Study the drawing (mm; zero at the part's minimum x, y, z) and answer. A direction names the side the tool comes from. Coordinates: 2 decimals unless noted, no trailing zeros. Order: outer loops, then holes, each group sorted by start corner. A loop starts at its lowest first (then second) coordinate and runs counter-clockwise, first axis right, second up.
1. A tool of negligible diameter and unlimited length cuts with its end or side. For the marked faces 1, 2, 3 and 4, from which of +Z, -Z, +X, -X, +Y, -Y can it reach the whole face along a straight path? Write none if from no direction.
2. The part is cut by section C-C, the plane x = 22. Give the vertices of the cut face in (y, z).
3. The part is cut by section A-A, the plane y = 2.5. Give the vertices of the cut face in (x, z), then the cut area to 3 significant figures.
4. Find the intervals of material crossed by probe 1 along X at (y, z) = (1.15, 25); probe 2 along Z at (x, y) = (10.05, 11), in increasing order.
5. Flat-ended cylindrical pins translate along their axes: pin 1 Ø8 at (x, y) = (27, 12.5) entering from -Z; pin 2 Ø2 at (x, y) = (5.5, 9.5) entering from +Z; pin 3 Ø2 at (y, z) = (10.5, 15.5) entering from +X. Find the tip coordinate at first contact, or state that the pin passes through.
6. The part is cut by section B-B, the plane z = 25. Give the vertices of the cut face in (x, y).
7. The part is cut by section D-D, the plane z = 18.5. Give the vertices of the cut face in (x, y).
8. Determine the mould class of the marked faces 5, 6, 7 and 8 for opening direction X: +X half, -X half, draft (parallel to the pull), parting line (faces both ways), or undercut.
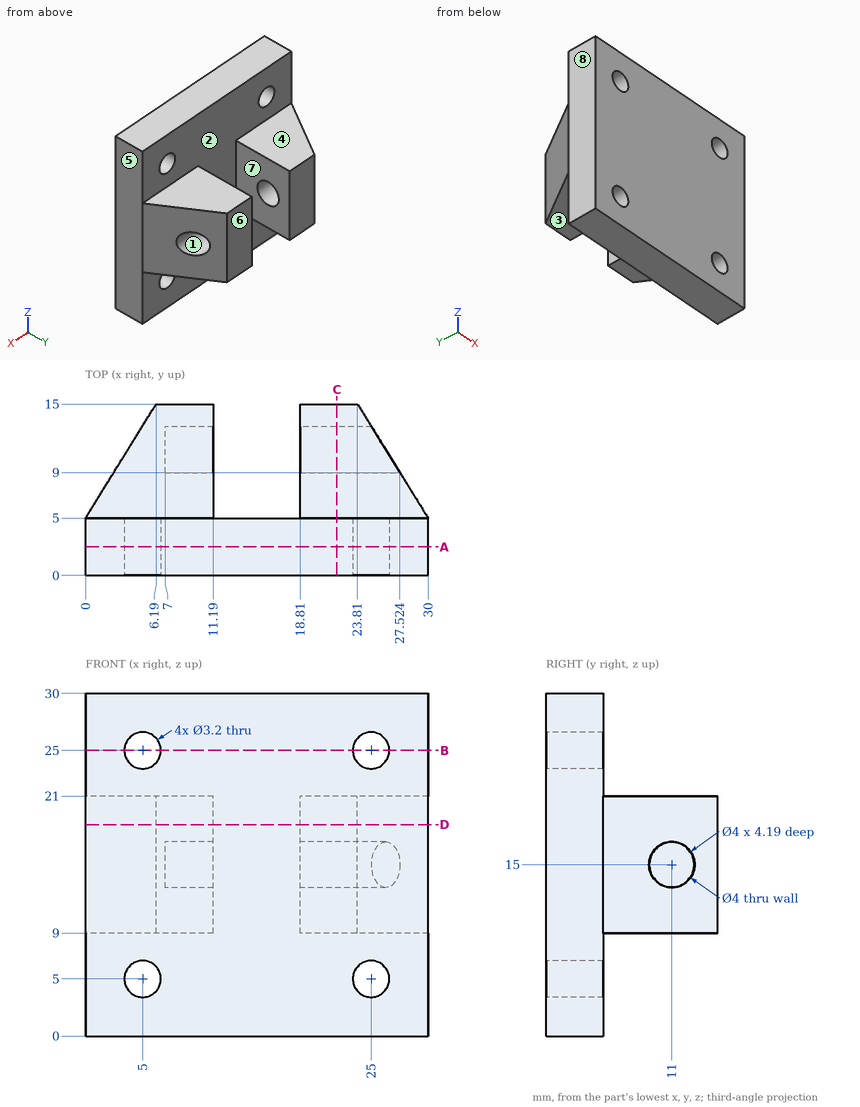
Geometry says:
1. face 1: +X
1. face 2: +Y
1. face 3: -Z, +X, -X, +Y
1. face 4: +Z, +X, -X, +Y
2. outline: (0, 0) - (5, 0) - (5, 9) - (15, 9) - (15, 21) - (5, 21) - (5, 30) - (0, 30) - close; hole circle Ø4 at (11, 15)
3. outline: (0, 0) - (30, 0) - (30, 30) - (0, 30) - close; hole circle Ø3.2 at (5, 5); hole circle Ø3.2 at (5, 25); hole circle Ø3.2 at (25, 5); hole circle Ø3.2 at (25, 25)
3. area: 868 mm2
4. probe 1: x = 0 to 3.4, 6.6 to 23.4, 26.6 to 30
4. probe 2: z = 9 to 13, 17 to 21
5. pin 1: stops at z = 9
5. pin 2: stops at z = 21
5. pin 3: stops at x = 7
6. outline: (0, 0) - (3.4, 0) - (3.4, 5) - (0, 5) - close; (6.6, 0) - (23.4, 0) - (23.4, 5) - (6.6, 5) - close; (26.6, 0) - (30, 0) - (30, 5) - (26.6, 5) - close
7. outline: (0, 0) - (30, 0) - (30, 5) - (23.81, 15) - (18.81, 15) - (18.81, 5) - (11.19, 5) - (11.19, 15) - (6.19, 15) - (0, 5) - close
8. face 5: +X half
8. face 6: draft
8. face 7: undercut
8. face 8: -X half
